For this review, use the dimensioned drawing (mm, ordinates from the lowest corner) and the shaded views. Give positions to 0.01 mm unless a question says otherwise; leave off trailing zeros. Order: outer loops, then holes, each group sorted by start corner. A loop starts at its lowest first (then second) coordinate and runs counter-clockwise, first axis right, second up. Notation, with made-up numbers: M 74.25,49 L 110.25,49 A17 cw 110.25,75 Z; hole C 52.25,-18.75 d4. An arc over 180 degrees is marked long. Use CSV: the item, a comma, the result in double quotes. Start each with the question number.
(1) Clearance check with a flat-ended pin moving along its axis: P1, Ø6, axis at x = 24.5, z = 20.5, coming from the -Y side. State where the tip first meets the part, or that it passes through.
(2) Wall thickness on L1, parallel to X at y = 0.5, z = 50.5; L2, parallel to Z at x = 27.5, y = 0.2; L3, parallel to X at y = 0.15, z = 11: over which ranges is each line inside the solid? List them lowest first. Write a range as from..to.
(3) Consider section A-A (z = 2). Write out the cut boundary in (x, y).
(4) Consider section D-D (z = 51). Write out the cut boundary in (x, y).
(5) Consider section C-C (x = 23.75). Write out the cut boundary in (y, z), and give its area (3 significant figures).
(6) Consider section B-B (y = 0.5). Write out the cut boundary in (x, z), and give its area (3 significant figures).
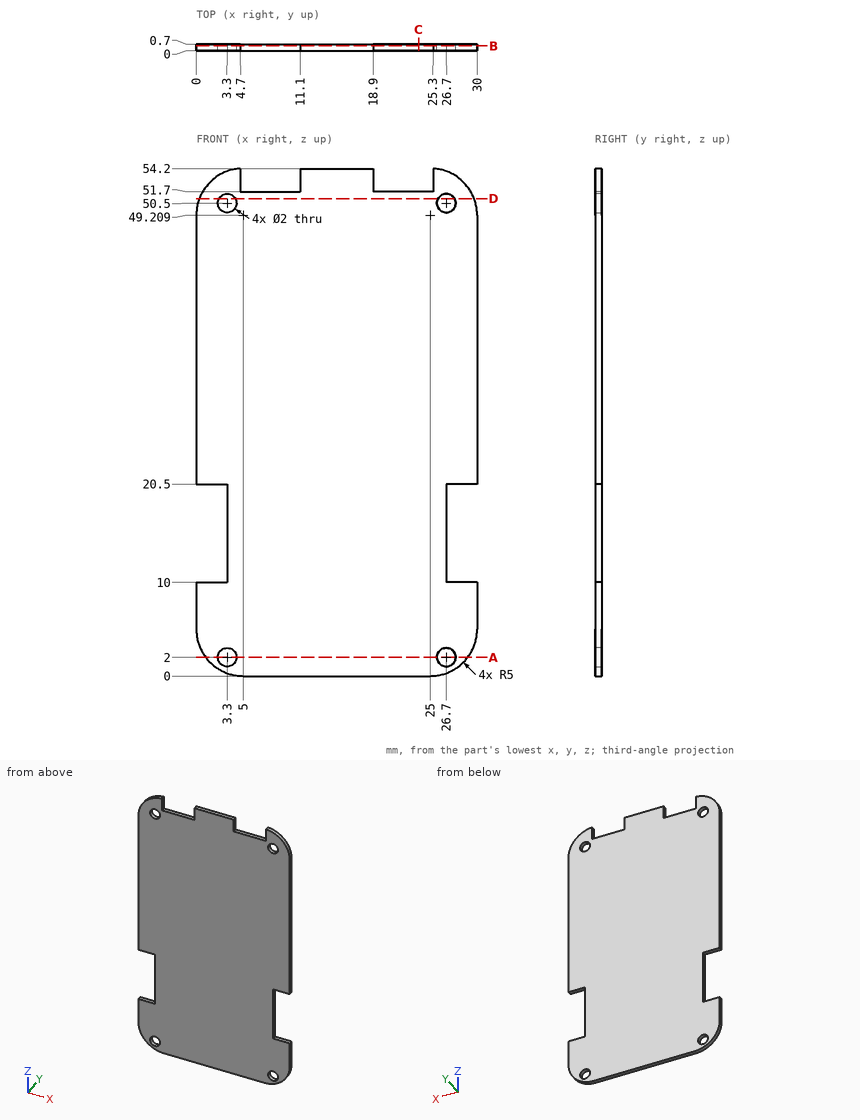
Check result:
1,P1,"stops at y = 0"
2,L1,"x = 0.17..2.3, 4.3..25.7, 27.7..29.83"
2,L2,"z = 0.67..1.4, 2.6..10, 20.5..49.9, 51.1..53.54"
2,L3,"x = 3.3..26.7"
3,outline,"M 1,0 L 2.3,0 L 2.3,0.7 L 1,0.7 Z; M 4.3,0 L 25.7,0 L 25.7,0.7 L 4.3,0.7 Z; M 27.7,0 L 29,0 L 29,0.7 L 27.7,0.7 Z"
4,outline,"M 0.33,0 L 2.43,0 L 2.43,0.7 L 0.33,0.7 Z; M 4.17,0 L 25.83,0 L 25.83,0.7 L 4.17,0.7 Z; M 27.57,0 L 29.67,0 L 29.67,0.7 L 27.57,0.7 Z"
5,outline,"M 0,0 L 0.7,0 L 0.7,51.7 L 0,51.7 Z"
5,area,"36.2 mm^2"
6,outline,"M 0,5 A5 ccw 5,0 L 25,0 A5 ccw 30,5 L 30,10 L 26.7,10 L 26.7,20.5 L 30,20.5 L 30,49.21 A5 ccw 25.3,54.2 L 25.3,51.7 L 18.9,51.7 L 18.9,54.2 L 11.1,54.2 L 11.1,51.7 L 4.7,51.7 L 4.7,54.2 A5 ccw 0,49.21 L 0,20.5 L 3.3,20.5 L 3.3,10 L 0,10 Z; hole C 3.3,2 d2; hole C 3.3,50.5 d2; hole C 26.7,2 d2; hole C 26.7,50.5 d2"
6,area,"1,490 mm^2"
